```python
from build123d import *

# Parameters (mm, degrees)
SKETCH268_R     = 4
PAD107_DEPTH    = 9.5
SKETCH269_R     = 3.85
SKETCH269_R_2   = 1.95
PAD108_DEPTH    = 2
SKETCH270_R     = 1.5
POCKET131_DEPTH = 4.001


with BuildPart() as part:
    # Sketch268 → Pad107 (new body)
    with BuildSketch(Plane.XY):
        Circle(SKETCH268_R)
        with BuildLine():
            Line((-1.245994, 1.5), (1.245994, 1.5))
            ThreePointArc((-1.245994, 1.5), (0, -1.95), (1.245994, 1.5))
        make_face(mode=Mode.SUBTRACT)
    extrude(amount=PAD107_DEPTH)

    # Sketch269 (on Face5 of Pad107) → Pad108 (join)
    with BuildSketch(Plane.XY.offset(9.5)):
        Circle(SKETCH269_R)
        Circle(SKETCH269_R_2, mode=Mode.SUBTRACT)
    extrude(amount=PAD108_DEPTH)

    # Sketch270 → Pocket131 (cut, through all)
    with BuildSketch(Plane.XZ):
        with Locations((0, 2.5)):
            Circle(SKETCH270_R)
    extrude(amount=-POCKET131_DEPTH, mode=Mode.SUBTRACT)


solid = part.part
```
Geometry: final body of the model. Coordinates: model frame, mm. A direction names the side the tool comes from. Round coordinates to 2 decimals unless told otherwise and drop trailing zeros. Loops run counter-clockwise (first coordinate to the right, second up) from the corner with the lowest first, then second, coordinate; pieces in that order, holes last. Notation, with made-up numbers: (13.25, 65) -> (41.25, 65) arc R18 ccw to (41.25, 80) -> close; hole circle Ø8 at (-21, -32). An arc over 180 degrees is marked (long way). Write each question's results on one line, items separated by ' | '.
Item 1: Line query: probe 1 along Y at (x, z) = (0, 7); probe 2 along Z at (x, y) = (0, 3.2); probe 3 along Y at (x, z) = (1, 4.75). Output: solid intervals per line, ascending. Write a range as [from, to].
Answers below:
probe 1: y = [-4, -1.95], [1.5, 4] | probe 2: z = [0, 1], [4, 11.5] | probe 3: y = [-3.87, -1.67], [1.5, 3.87]
Item 2: Set-up query: faces 1 (the face through (1.43, 2.6, 2.95)), 2 (the face through (-2, 1, 11.5)). Return all of +Z, -Z, +X, -X, +Y, -Y with unobstructed straight access to the full face (end or side cutting, diameter ignored); none if empty.
Answers below:
face 1: +Y | face 2: +Z, +X, -X, +Y, -Y
Item 3: Cut plane D-D on y = 3.5. Return the cut outline in (x, z), and give its area (3 significant figures).
Answers below:
outline: (-1.94, 0) -> (1.94, 0) -> (1.94, 9.5) -> (1.6, 9.5) -> (1.6, 11.5) -> (-1.6, 11.5) -> (-1.6, 9.5) -> (-1.94, 9.5) -> close; hole circle Ø3 at (0, 2.5) | area: 36.1 mm²
Item 4: Pin query (flat end, axial travel): pin 1 Ø2 at (y, z) = (-3, 7) entering from -X. Return the tip coordinate at first contact, or that it passes through.
Answers below:
pin 1: stops at x = -3.46
Item 5: Pull-direction query (Y, two-part tool) for faces 3 (the face through (0, 1.5, 6)), 4 (the face through (0, 2, 0)), 5 (the face through (0, 1.5, 0.6)), 6 (the face through (-0.83, -3.76, 10.49)); classes: pulls with the +Y half, pulls with the -Y half, needs draft (parallel to the pull), parting line crosses it, or undercut.
Answers below:
face 3: undercut | face 4: needs draft | face 5: undercut | face 6: parting line crosses it
Item 6: Cut plane C-C on z = 4.5. Return the cut outline in (x, y).
Answers below:
outline: circle Ø8 at (0, 0); hole (-1.25, 1.5) arc R1.95 ccw (long way) to (1.25, 1.5) -> close
Item 7: Cut plane A-A on y = 0. Return the cut outline in (x, z).
Answers below:
outline: (-4, 0) -> (-1.95, 0) -> (-1.95, 11.5) -> (-3.85, 11.5) -> (-3.85, 9.5) -> (-4, 9.5) -> close; (1.95, 0) -> (4, 0) -> (4, 9.5) -> (3.85, 9.5) -> (3.85, 11.5) -> (1.95, 11.5) -> close
Item 8: Cut plane B-B on x = 0. Return the cut outline in (y, z).
Answers below:
outline: (-4, 0) -> (-1.95, 0) -> (-1.95, 11.5) -> (-3.85, 11.5) -> (-3.85, 9.5) -> (-4, 9.5) -> close; (1.5, 0) -> (4, 0) -> (4, 1) -> (1.5, 1) -> close; (1.5, 4) -> (4, 4) -> (4, 9.5) -> (3.85, 9.5) -> (3.85, 11.5) -> (1.95, 11.5) -> (1.95, 9.5) -> (1.5, 9.5) -> close
